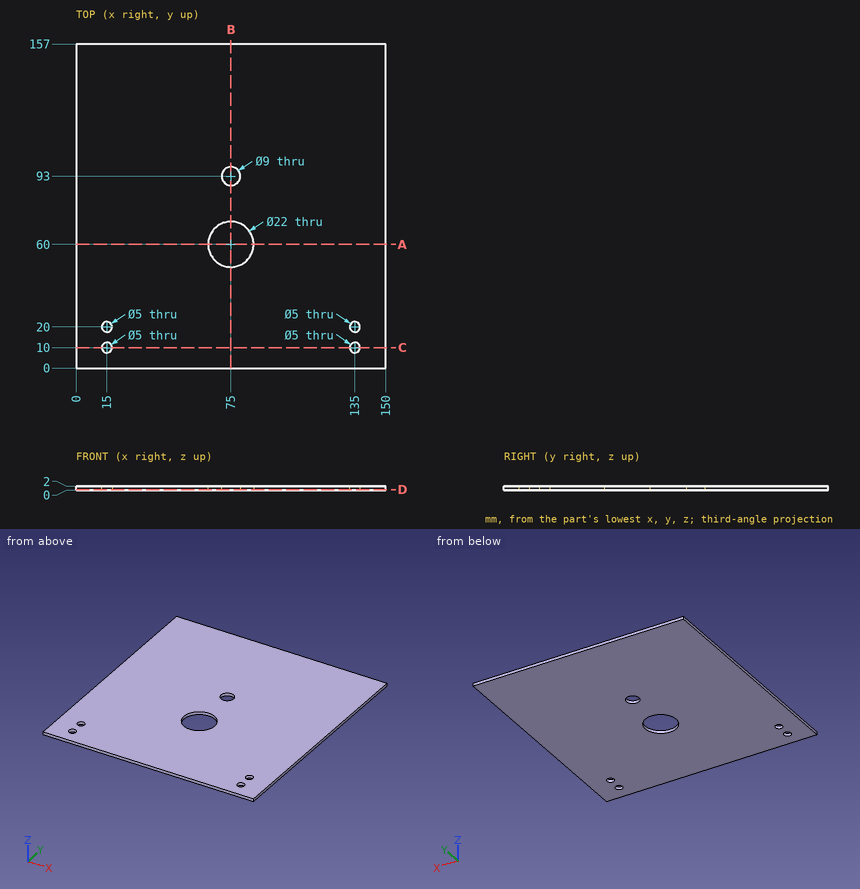
Check sheet for the drawn part. Datum: minimum x, y, z corner. Units: mm. Round coordinates to 2 decimals unless told otherwise and drop trailing zeros. Order: outer loops, then holes, each group sorted by start corner. A loop starts at its lowest first (then second) coordinate and runs counter-clockwise, first axis right, second up. Notation, with made-up numbers: (22, 16.5) -> (56, 16.5) arc R19 cw to (56, 53.5) -> close; hole circle Ø8 at (-5.75, -19.5). An arc over 180 degrees is marked (long way). Put each result on its own line as item: value. Start each with the question number.
(1) Section check B-B (x = 75). Enter the section's corners in (y, z).
(2) Depth check by flat-ended pin: pin 1 Ø5.5 at (x, y) = (75, 93) entering from +Z. Enter the tip coordinate at first touch or a pass-through.
(3) Section check C-C (y = 10). Enter the section's corners in (x, z), then the cut area to 3 significant figures.
(4) Section check A-A (y = 60). Enter the section's corners in (x, z).
(5) Material ranges on line 1 along Y through (x, z) = (75, 1.4); line 2 along Y through (x, z) = (135, 1.4), recorded low to high.
(6) Section check D-D (z = 0.35). Enter the section's corners in (x, y), then the cut area to 3 significant figures.
Completed:
1. outline: (0, 0) -> (49, 0) -> (49, 2) -> (0, 2) -> close; (71, 0) -> (88.5, 0) -> (88.5, 2) -> (71, 2) -> close; (97.5, 0) -> (157, 0) -> (157, 2) -> (97.5, 2) -> close
2. pin 1: passes through
3. outline: (0, 0) -> (12.5, 0) -> (12.5, 2) -> (0, 2) -> close; (17.5, 0) -> (132.5, 0) -> (132.5, 2) -> (17.5, 2) -> close; (137.5, 0) -> (150, 0) -> (150, 2) -> (137.5, 2) -> close
3. area: 280 mm2
4. outline: (0, 0) -> (64, 0) -> (64, 2) -> (0, 2) -> close; (86, 0) -> (150, 0) -> (150, 2) -> (86, 2) -> close
5. line 1: y = 0 to 49, 71 to 88.5, 97.5 to 157
5. line 2: y = 0 to 7.5, 12.5 to 17.5, 22.5 to 157
6. outline: (0, 0) -> (150, 0) -> (150, 157) -> (0, 157) -> close; hole circle Ø5 at (15, 10); hole circle Ø5 at (15, 20); hole circle Ø22 at (75, 60); hole circle Ø9 at (75, 93); hole circle Ø5 at (135, 10); hole circle Ø5 at (135, 20)
6. area: 23,000 mm2
